The model under review builds one solid part; all positions refer to its coordinate system, in mm. Give positions to 0.01 mm unless a question says otherwise; leave off trailing zeros. Loops run counter-clockwise (first coordinate to the right, second up) from the corner with the lowest first, then second, coordinate; pieces in that order, holes last. Notation, with made-up numbers: M 87,2 L 134,2 A23 ccw 134,24 Z; hole C 70,59 d5. An arc over 180 degrees is marked long. Put each result on its own line as item: value. Start each with the question number.
Autodesk Inventor part; units mm, degrees
ref_plane "YZ Plane" through (0, 0, 0) normal (1, 0, 0) x (0, 1, 0)
ref_plane "XZ Plane" through (0, 0, 0) normal (0, 1, 0) x (-1, 0, 0)
ref_plane "XY Plane" through (0, 0, 0) normal (0, 0, 1) x (1, 0, 0)
sketch "Sketch1" plane through (0, 0, 0) normal (0, 0, 1) x (1, 0, 0)
  line L0 (-2.3, 0) -> (-3, 0)
  line L1 (-3, 0) -> (-3, 38)
  line L2 (-3, 38) -> (-2.3, 38)
  line L3 (-2.3, 38) -> (-2.3, 0)
  line L4 (0, 0) -> (0, 38)
  point P0 (-2.65, 38)
  point P1 (-2.65, 0)
  dimension "d0" = 0.7
  dimension "d1" = 6
  dimension "d2" = 38
revolve "Revolution1" add sketch "Sketch1" angle 330 about axis through (0, 0, 0) along (0, 1, 0)
chamfer "Chamfer1" distance 0.5 angle 60 1 edges at (2.8978, 38, 0.7765) measured on face at (-0.4754, 38, -2.7069)
chamfer "Chamfer2" distance 0.5 angle 60 1 edges at (2.8978, 0, 0.7765) measured on face at (1.8107, 0, -2.0675)
Item 1: Draft analysis for pull direction Z (two halves, no side actions). For faces 1 (the conical face through (2.524, 37.85, 0.568)), 2 (the cylindrical face through (2.244, 18.734, 0.505)), state which applies: +Z half, -Z half, draft (parallel to the pull), parting line (faces both ways), or undercut.
Item 2: To check wall thickness, follow L1, parallel to Z at x = 0, y = 14.5; L2, parallel to Z at x = 2.05, y = 22.5. State the ranges of each line that lie inside material, in increasing order. Write a range as [from, to].
Item 3: Consider section B-B, the plane y = 25. Write out the cut boundary in (x, z), plus the area to 3 significant figures.
Item 4: Consider section A-A, the plane x = 0. Write out the cut boundary in (y, z), plus the area to 3 significant figures.
Item 5: Clearance check with a flat-ended pin moving along its axis: pin 1 Ø2 at (x, z) = (2, 2) entering from -Y. State where the tip first meets the part, or that it passes through.
Report:
1. face 1: parting line
1. face 2: undercut
2. L1: [-3, -2.3], [2.3, 3]
2. L2: [-2.19, -1.04], [1.04, 2.19]
3. outline: M -3,0 L -2.3,0 A2.3 cw long -1.99,-1.15 L -2.6,-1.5 A3 ccw long Z
3. area: 10.7 mm²
4. outline: M 0,-2.5 L 0.87,-3 L 37.13,-3 L 38,-2.5 L 38,-2.3 L 0,-2.3 Z; M 0,2.3 L 38,2.3 L 38,2.5 L 37.13,3 L 0.87,3 L 0,2.5 Z
4. area: 52.3 mm²
5. pin 1: y = 0
